from build123d import *

# Parameters (mm, degrees)
PAD_DEPTH    = 7.3
POCKET_DEPTH = 6


with BuildPart() as part:
    # Sketch → Pad (new body)
    with BuildSketch(Plane.XZ):
        with BuildLine():
            ThreePointArc((-3.47, 3.26), (-4.177107, 2.967107), (-4.47, 2.26))
            Line((-4.47, 2.26), (-4.47, 1))
            ThreePointArc((-4.47, 1), (-4.177107, 0.292893), (-3.47, 0))
            Line((3.47, 0), (-3.47, 0))
            ThreePointArc((3.47, 0), (4.177107, 0.292893), (4.47, 1))
            Line((4.47, 2.26), (4.47, 1))
            ThreePointArc((4.47, 2.26), (4.177107, 2.967107), (3.47, 3.26))
            Line((-3.47, 3.26), (3.47, 3.26))
        make_face()
    extrude(amount=PAD_DEPTH)

    # Sketch001 (on Face10 of Pad) → Pocket (cut)
    with BuildSketch(Plane.XZ.offset(7.3)):
        with BuildLine():
            ThreePointArc((-3.47, 2.96), (-3.964975, 2.754975), (-4.17, 2.26))
            Line((-4.17, 2.26), (-4.17, 1))
            ThreePointArc((-4.17, 1), (-3.964975, 0.505025), (-3.47, 0.3))
            Line((-3.47, 0.3), (3.47, 0.3))
            ThreePointArc((3.47, 0.3), (3.964975, 0.505025), (4.17, 1))
            Line((4.17, 1), (4.17, 2.26))
            ThreePointArc((4.17, 2.26), (3.964975, 2.754975), (3.47, 2.96))
            Line((-3.47, 2.96), (3.47, 2.96))
        make_face()
        with BuildLine():
            ThreePointArc((-3.47, 2.46), (-3.611421, 2.401421), (-3.67, 2.26))
            Line((-3.67, 2.26), (-3.67, 1))
            ThreePointArc((-3.67, 1), (-3.611421, 0.858579), (-3.47, 0.8))
            Line((-3.47, 0.8), (3.47, 0.8))
            ThreePointArc((3.47, 0.8), (3.61212, 0.859281), (3.66999, 1.001982))
            Line((3.66999, 1.001982), (3.66999, 2.261982))
            ThreePointArc((3.66999, 2.261982), (3.610719, 2.40212), (3.47, 2.46))
            Line((-3.47, 2.46), (3.47, 2.46))
        make_face(mode=Mode.SUBTRACT)
    extrude(amount=-POCKET_DEPTH, mode=Mode.SUBTRACT)


solid = part.part
CAD build for the part. Positions are in the model's coordinates, mm. A direction names the side the tool comes from. Give positions to 0.01 mm unless a question says otherwise; leave off trailing zeros. Loops run counter-clockwise (first coordinate to the right, second up) from the corner with the lowest first, then second, coordinate; pieces in that order, holes last. Notation, with made-up numbers: M 14,-10.5 L 31,-10.5 A19 cw 31,4.5 Z; hole C -15.5,13.5 d11. An arc over 180 degrees is marked long. Answer in a Markdown table with one row per item. Add a question column.
Item 1: Band-saw the part on D-D on y = -0.25. Give the cut face in (x, z).
Item 2: Band-saw the part on C-C on z = 1.85. Give the cut face in (x, y).
Item 3: Band-saw the part on B-B on x = -2.5. Give the cut face in (y, z).
Item 4: Tool access for faces 5 (the face through (0, -4, 0.3)), 6 (the face through (-4.47, -4, 2)): list every direction of +Z, -Z, +X, -X, +Y, -Y with a clear straight run to the whole face (end or side of a thin tool).
Item 5: Mould opens along X. For faces 1 (the face through (-4.185, -3.599, 0.301)), 2 (the face through (4.185, -3.599, 2.959)), 3 (the face through (-0.1, -1.3, 2.8)), 4 (the face through (0, -4, 3.26)) say: +X half, -X half, draft (parallel to the pull), parting line (faces both ways), or undercut.
Item 6: Band-saw the part on A-A on y = -5. Give the cut face in (x, z), then the cut area to 3 significant figures.
Item 7: Probe probe 1 along Z at (x, y) = (2.25, -1.5); probe 2 along X at (y, z) = (-2.5, 1.5); probe 3 along X at (y, z) = (-6, 2.35). List the from-to ranges inside material, lowest first.
Reply:
| question | item | result |
|---|---|---|
| 1 | outline | M -4.47,1 A1 ccw -3.47,0 L 3.47,0 A1 ccw 4.47,1 L 4.47,2.26 A1 ccw 3.47,3.26 L -3.47,3.26 A1 ccw -4.47,2.26 Z |
| 2 | outline | M -4.47,-7.3 L -4.17,-7.3 L -4.17,-1.3 L -3.67,-1.3 L -3.67,-7.3 L 3.67,-7.3 L 3.67,-1.3 L 4.17,-1.3 L 4.17,-7.3 L 4.47,-7.3 L 4.47,0 L -4.47,0 Z |
| 3 | outline | M -7.3,0 L 0,0 L 0,3.26 L -7.3,3.26 L -7.3,2.96 L -1.3,2.96 L -1.3,2.46 L -7.3,2.46 L -7.3,0.8 L -1.3,0.8 L -1.3,0.3 L -7.3,0.3 Z |
| 4 | face 5 | -Y |
| 4 | face 6 | +Z, -Z, -X, +Y, -Y |
| 5 | face 1 | -X half |
| 5 | face 2 | +X half |
| 5 | face 3 | undercut |
| 5 | face 4 | draft |
| 6 | outline | M -4.47,1 A1 ccw -3.47,0 L 3.47,0 A1 ccw 4.47,1 L 4.47,2.26 A1 ccw 3.47,3.26 L -3.47,3.26 A1 ccw -4.47,2.26 Z; M -3.67,1 A0.2 ccw -3.47,0.8 L 3.47,0.8 A0.2 ccw 3.67,1 L 3.67,2.26 A0.2 ccw 3.47,2.46 L -3.47,2.46 A0.2 ccw -3.67,2.26 Z; hole M -4.17,1 A0.7 ccw -3.47,0.3 L 3.47,0.3 A0.7 ccw 4.17,1 L 4.17,2.26 A0.7 ccw 3.47,2.96 L -3.47,2.96 A0.7 ccw -4.17,2.26 Z |
| 6 | area | 18.7 mm^2 |
| 7 | probe 1 | z = 0 to 0.3, 0.8 to 2.46, 2.96 to 3.26 |
| 7 | probe 2 | x = -4.47 to -4.17, -3.67 to 3.67, 4.17 to 4.47 |
| 7 | probe 3 | x = -4.47 to -4.16, -3.65 to 3.65, 4.16 to 4.47 |
